Job drawing, mm, ordinate dimensions from the low corner. One solid piece. A direction names the side the tool comes from. Round coordinates to 2 decimals unless told otherwise and drop trailing zeros. Order: outer loops, then holes, each group sorted by start corner. A loop starts at its lowest first (then second) coordinate and runs counter-clockwise, first axis right, second up. Notation, with made-up numbers: (56.25, -28.5) -> (105.25, -28.5) arc R22 cw to (105.25, -9.5) -> close; hole circle Ø4 at (42, 15.25). An arc over 180 degrees is marked (long way). Write item = value, one per line.
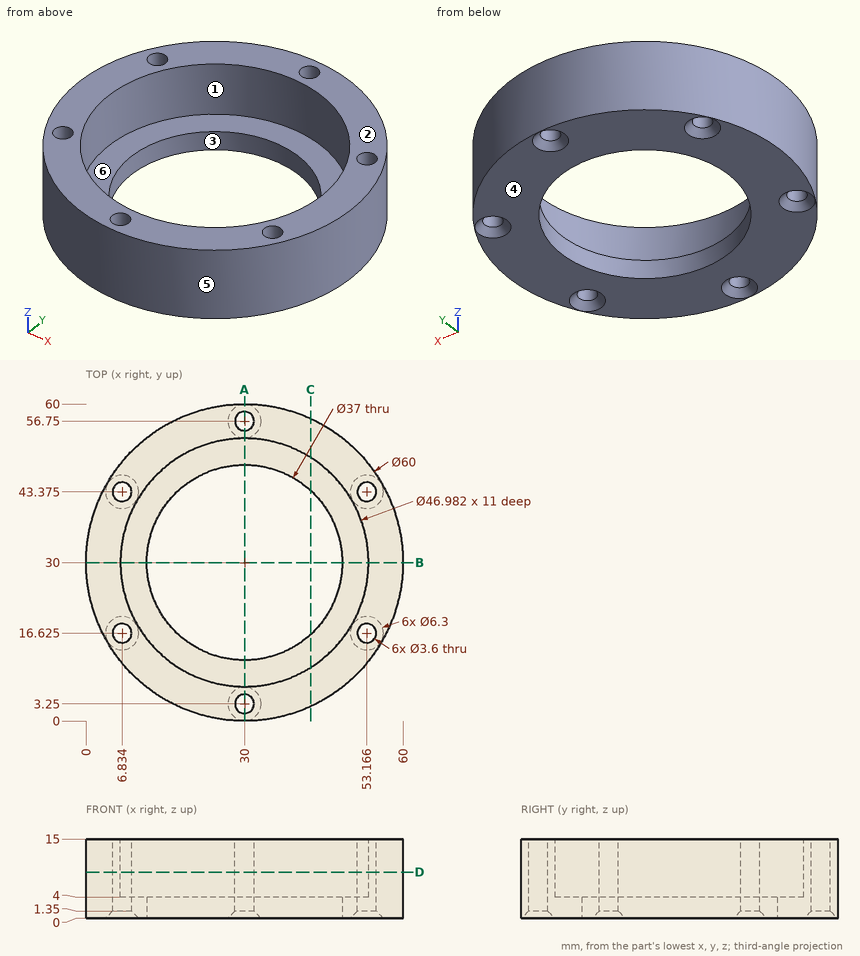
Q1. Mould opens along Y. For the marked faces 3, 4, 5 and 6 say: released by +Y, released by -Y, zero draft, split by the parting line, or undercut.
Check values:
face_3 = undercut
face_4 = zero draft
face_5 = split by the parting line
face_6 = undercut
Q2. Cut at C-C, the plane x = 42.5. List the corners of the cut face in (y, z).
Check values:
outline = (2.73, 0) -> (16.36, 0) -> (16.36, 4) -> (10.11, 4) -> (10.11, 15) -> (2.73, 15) -> close; (43.64, 0) -> (57.27, 0) -> (57.27, 15) -> (49.89, 15) -> (49.89, 4) -> (43.64, 4) -> close
Q3. Which spindle directions (+Z, -Z, +X, -X, +Y, -Y) get a long thin tool onto all of the face, cutting with end or side? Do the marked faces 1 and 2. Say none if no direction does.
Check values:
face_1 = +Z
face_2 = +Z, +X, -X, +Y, -Y
Q4. Cut at A-A, the plane x = 30. List the corners of the cut face in (y, z).
Check values:
outline = (0, 0) -> (0.1, 0) -> (1.45, 1.35) -> (1.45, 15) -> (0, 15) -> close; (5.05, 1.35) -> (6.4, 0) -> (11.5, 0) -> (11.5, 4) -> (6.51, 4) -> (6.51, 15) -> (5.05, 15) -> close; (48.5, 0) -> (53.6, 0) -> (54.95, 1.35) -> (54.95, 15) -> (53.49, 15) -> (53.49, 4) -> (48.5, 4) -> close; (58.55, 1.35) -> (59.9, 0) -> (60, 0) -> (60, 15) -> (58.55, 15) -> close
Q5. Cut at B-B, the plane y = 30. List the corners of the cut face in (x, z).
Check values:
outline = (0, 0) -> (11.5, 0) -> (11.5, 4) -> (6.51, 4) -> (6.51, 15) -> (0, 15) -> close; (48.5, 0) -> (60, 0) -> (60, 15) -> (53.49, 15) -> (53.49, 4) -> (48.5, 4) -> close
Q6. Probe probe 1 along Y at (x, z) = (30, 4.75); probe 2 along Y at (x, z) = (6, 11.5); probe 3 along X at (y, z) = (44, 13.75) (1 decimal). List the from-to ranges inside material, lowest first.
Check values:
probe_1 = 0 to 1.45, 5.05 to 6.51, 53.49 to 54.95, 58.55 to 60
probe_2 = 12 to 15.03, 18.22 to 41.78, 44.97 to 48
probe_3 = 3.5 to 5.1, 8.5 to 11.1, 48.9 to 51.5, 54.9 to 56.5
Q7. Flat gauge pins, fed straight in: pin 1 (6 mm diameter, centred on x = 53.17, y = 16.62, fed in from +Z); pin 2 (1.5 mm diameter, centred on x = 8, z = 6, fed in from -Y) (1 decimal); pin 3 (4 mm diameter, centred on x = 10, z = 3, fed in from -Y); pin 4 (4 mm diameter, centred on y = 26, z = 12.5, fed in from +X). Where does each tip first touch, or does it go through?
Check values:
pin_1 = 15
pin_2 = 8.8
pin_3 = 6
pin_4 = 59.93
Q8. Cut at D-D, the plane z = 8.75. Give the number of separate pieces and of enclosed holes in the cut face, and give its area (3 significant figures).
Check values:
separate_pieces = 1
enclosed_holes = 7
area = 1,030 mm²
